Build history of the part. All positions in model axes, mm. A direction names the side the tool comes from. Give positions to 0.01 mm unless a question says otherwise; leave off trailing zeros. Write each loop counter-clockwise with the first axis right and the second up, starting at its lowest first coordinate (ties: lowest second). Pieces come first, ordered by that corner, then holes. Notation, with made-up numbers: (12, 43.25) -> (41, 43.25) arc R31 cw to (41, 80.25) -> close; hole circle Ø2 at (59.5, 30.25). An arc over 180 degrees is marked (long way). Put each result on its own line as item: value.
from build123d import *

# Parameters (mm, degrees)
SKETCH1_R               = 2.25
SKETCH1_R_2             = 9.5
SKETCH1_R_3             = 7.5
BOSS_EXTRUDE1_DEPTH     = 24
SKETCH2_W               = 34
SKETCH2_H               = 33
CUT_EXTRUDE1_DEPTH      = 15
CUT_EXTRUDE2_DEPTH      = 59
CUT_EXTRUDE2_DEPTH_BACK = 23
FILLET1_R               = 3


with BuildPart() as part:
    # Sketch1 → Boss-Extrude1 (new body)
    with BuildSketch(Plane(origin=(0, 0, 0), x_dir=(1, 0, 0), z_dir=(0, 1, 0))):
        with BuildLine():
            Line((21, 11.832159566), (21, 66.5))
            Line((21, 66.5), (-21, 66.5))
            Line((-21, 66.5), (-21, 9.486832981))
            ThreePointArc((-21, 9.486832981), (-37.673494975, -5.361902647), (-16, 0))
            Line((-16, 0), (-16, 29.5))
            Line((-16, 29.5), (14, 29.5))
            Line((14, 29.5), (14, 0))
            ThreePointArc((14, 0), (39.118950039, -6.873863542), (21, 11.832159566))
        make_face()
        with Locations((-11, 38.5)):
            Circle(SKETCH1_R, mode=Mode.SUBTRACT)
        with Locations((-11, 61.5)):
            Circle(SKETCH1_R, mode=Mode.SUBTRACT)
        with Locations((11, 61.5)):
            Circle(SKETCH1_R, mode=Mode.SUBTRACT)
        with Locations((11, 38.5)):
            Circle(SKETCH1_R, mode=Mode.SUBTRACT)
        with Locations((27.5, 0)):
            Circle(SKETCH1_R_2, mode=Mode.SUBTRACT)
        with Locations((-27.5, 0)):
            Circle(SKETCH1_R_3, mode=Mode.SUBTRACT)
    extrude(amount=BOSS_EXTRUDE1_DEPTH)

    # Sketch2 → Cut-Extrude1 (cut)
    with BuildSketch(Plane(origin=(0, 24, 0), x_dir=(1, 0, 0), z_dir=(0, 1, 0))):
        with Locations((0, 50)):
            Rectangle(SKETCH2_W, SKETCH2_H)
    extrude(amount=-CUT_EXTRUDE1_DEPTH, mode=Mode.SUBTRACT)

    # Sketch4 → Cut-Extrude2 (cut, two sides)
    with BuildSketch(Plane(origin=(-17, 0, 0), x_dir=(0, 0, -1), z_dir=(1, 0, 0))) as cut_extrude2_sk:
        Polygon((33.5, 24), (66.5, 9), (66.5, 24), align=None)
    extrude(amount=CUT_EXTRUDE2_DEPTH, mode=Mode.SUBTRACT)
    extrude(cut_extrude2_sk.sketch, amount=-CUT_EXTRUDE2_DEPTH_BACK, mode=Mode.SUBTRACT)

    # Fillet1
    fillet1_edges = [part.edges().sort_by_distance(p)[0] for p in [
        (14, 12, -29.5),
        (-16, 12, -29.5),
        (-21, 12, -9.486832981),
        (21, 12, -11.832159566),
        (-17, 16.5, -33.5),
        (17, 16.5, -33.5),
        (-21, 4.5, -66.5),
        (21, 4.5, -66.5),
    ]]
    fillet(fillet1_edges, radius=FILLET1_R)


solid = part.part
1) Slice it at A-A (x = -27.5). Write the cut outline in (y, z), plus the area to 3 significant figures.
Filled sheet:
outline: (0, -11.5) -> (24, -11.5) -> (24, -7.5) -> (0, -7.5) -> close; (0, 7.5) -> (24, 7.5) -> (24, 11.5) -> (0, 11.5) -> close
area: 192 mm2
2) Slice it at C-C (z = -28). Write the cut outline in (x, y).
Filled sheet:
outline: (-21, 0) -> (-15.6, 0) -> (-15.6, 24) -> (-21, 24) -> close; (13.6, 0) -> (21, 0) -> (21, 24) -> (13.6, 24) -> close
3) Pin check, flat tips, straight feed: pin 1 (16.5 mm diameter, centred on x = -6, z = -55, fed in from +Y); pin 2 (9 mm diameter, centred on x = -27.5, z = 0, fed in from -Y); pin 3 (12 mm diameter, centred on y = 12, z = -13, fed in from -X); pin 4 (12 mm diameter, centred on x = 3.5, y = 17.5, fed in from -Z). Stop position of each tip, or through.
Filled sheet:
pin 1: y = 9
pin 2: through
pin 3: x = -36.62
pin 4: z = -33.5
4) Pull direction Z, two halves, no side cores. Call faces 1 (the cylindrical face through (-11.29, 4.44, -40.73)), 2 (the cylindrical face through (13.14, 12.17, -28.6)), 3 (the cylindrical face through (-20.1, 5.25, -65.64)), 4 (the flat face through (0, 9, -50)): released by +Z, released by -Z, zero draft, split by the parting line, or undercut.
Filled sheet:
face 1: undercut
face 2: released by +Z
face 3: released by -Z
face 4: zero draft
5) Slice it at B-B (x = -11). Write the cut outline in (y, z), plus the area to 3 significant figures.
Filled sheet:
outline: (0, -66.5) -> (9, -66.5) -> (9, -63.75) -> (0, -63.75) -> close; (0, -59.25) -> (9, -59.25) -> (9, -40.75) -> (0, -40.75) -> close; (0, -36.25) -> (9, -36.25) -> (9, -33.5) -> (24, -33.5) -> (24, -29.5) -> (0, -29.5) -> close
area: 312 mm2
6) Slice it at D-D (z = -61.5). Write the cut outline in (x, y), plus the area to 3 significant figures.
Filled sheet:
outline: (-21, 0) -> (-13.25, 0) -> (-13.25, 9) -> (-17, 9) -> (-17, 11.27) -> (-21, 11.27) -> close; (-8.75, 0) -> (8.75, 0) -> (8.75, 9) -> (-8.75, 9) -> close; (13.25, 0) -> (21, 0) -> (21, 11.27) -> (17, 11.27) -> (17, 9) -> (13.25, 9) -> close
area: 315 mm2
7) Tool access for faces 5 (the cylindrical face through (-15.1, 12.17, -28.64)), 6 (the flat face through (-17, 13, -45)), 7 (the flat face through (21, 9, -34)): list every direction of +Z, -Z, +X, -X, +Y, -Y with a clear straight run to the whole face (end or side of a thin tool).
Filled sheet:
face 5: +Z, +Y, -Y
face 6: -Z, +Y
face 7: -Z, +X, +Y, -Y
8) Wall check: L1, parallel to Z at x = 11, y = 4.25; L2, parallel to X at y = 5.75, z = -61.5; L3, parallel to X at y = 4, z = -19.5. Give the ranges that are in metal, low to high.
Filled sheet:
L1: -66.5 to -63.75, -59.25 to -40.75, -36.25 to -29.5
L2: -21 to -13.25, -8.75 to 8.75, 13.25 to 21
L3: -21 to -16, 14 to 21
